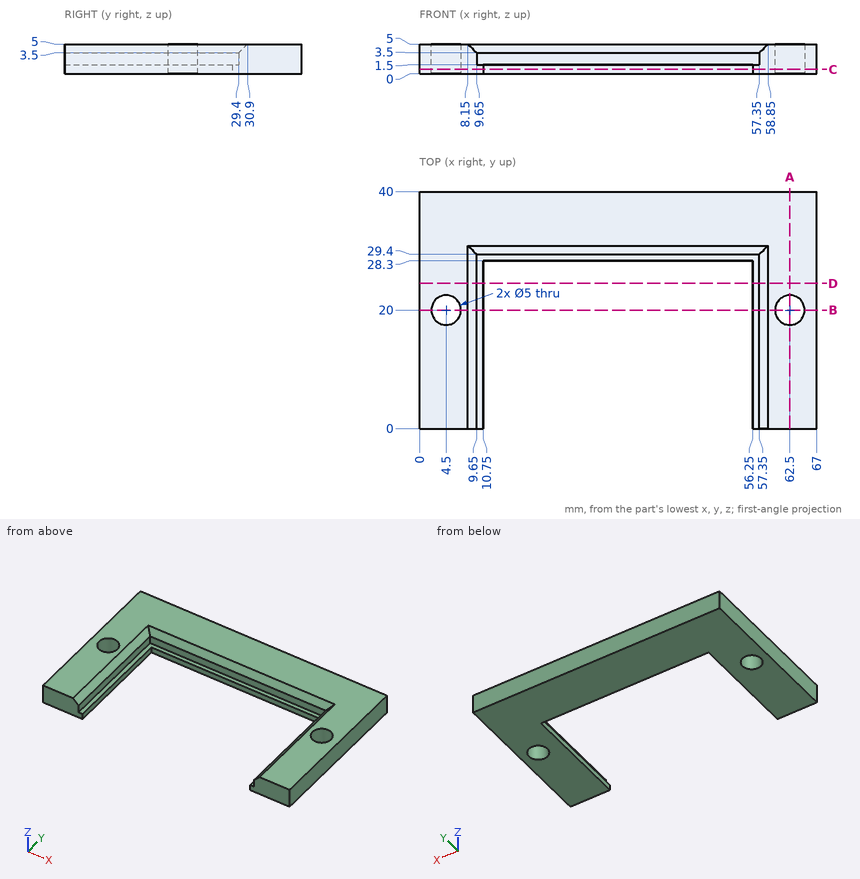
Here's the drawing with two shaded views (mm, measured from the low corner). I have some questions. Give positions to 0.01 mm unless a question says otherwise; leave off trailing zeros. Loops run counter-clockwise (first coordinate to the right, second up) from the corner with the lowest first, then second, coordinate; pieces in that order, holes last. Notation, with made-up numbers: (-15, 66) - (43, 66) arc R12 ccw to (43, 80) - close; hole circle Ø10 at (44, -23.5). An arc over 180 degrees is marked (long way). Return JSON: item names as keys, results as strings.
1. I'm going to push a flat-ended pin straight in: pin 1 Ø0.6 at (x, z) = (41, 2.5) entering from -Y. Where does the tip first touch, or does it pass through?
Output values:
{"pin 1": "stops at y = 29.4"}
2. If I drill on line 1 (X direction, y = 3.5, z = 2); line 2 (Y direction, x = 4.5, z = 1.1); line 3 (X direction, y = 9.5, z = 0.9), over which ranges is the centre line in solid material (lowest first)?
Output values:
{"line 1": "x = 0 to 9.65, 57.35 to 67", "line 2": "y = 0 to 17.5, 22.5 to 40", "line 3": "x = 0 to 10.75, 56.25 to 67"}
3. I want a section at B-B on y = 20. Please give me the cut outline in (x, z), and give its area (4 significant figures).
Output values:
{"outline": "(0, 0) - (2, 0) - (2, 5) - (0, 5) - close; (7, 0) - (10.75, 0) - (10.75, 1.5) - (9.65, 1.5) - (9.65, 3.5) - (8.15, 5) - (7, 5) - close; (56.25, 0) - (60, 0) - (60, 5) - (58.85, 5) - (57.35, 3.5) - (57.35, 1.5) - (56.25, 1.5) - close; (65, 0) - (67, 0) - (67, 5) - (65, 5) - close", "area": "47.55 mm²"}
4. I want a section at C-C on z = 0.7. Please give me the cut outline in (x, y), and give its area (3 significant figures).
Output values:
{"outline": "(0, 0) - (10.75, 0) - (10.75, 28.3) - (56.25, 28.3) - (56.25, 0) - (67, 0) - (67, 40) - (0, 40) - close; hole circle Ø5 at (4.5, 20); hole circle Ø5 at (62.5, 20)", "area": "1,350 mm²"}
5. I want a section at D-D on y = 24.5. Please give me the cut outline in (x, z), and give its area (4 significant figures).
Output values:
{"outline": "(0, 0) - (10.75, 0) - (10.75, 1.5) - (9.65, 1.5) - (9.65, 3.5) - (8.15, 5) - (0, 5) - close; (56.25, 0) - (67, 0) - (67, 5) - (58.85, 5) - (57.35, 3.5) - (57.35, 1.5) - (56.25, 1.5) - close", "area": "97.55 mm²"}
6. I want a section at A-A on x = 62.5. Please give me the cut outline in (y, z).
Output values:
{"outline": "(0, 0) - (17.5, 0) - (17.5, 5) - (0, 5) - close; (22.5, 0) - (40, 0) - (40, 5) - (22.5, 5) - close"}
